Check sheet for the modelled part. Datum: model origin and axes. Units: mm. A direction names the side the tool comes from. Give positions to 0.01 mm unless a question says otherwise; leave off trailing zeros. Write each loop counter-clockwise with the first axis right and the second up, starting at its lowest first coordinate (ties: lowest second). Pieces come first, ordered by that corner, then holes. Notation, with made-up numbers: (40.5, 23) -> (99.5, 23) arc R30 cw to (99.5, 59) -> close; hole circle Ø2 at (0, 32). An arc over 180 degrees is marked (long way). Return JSON: item names as keys, results as strings.
from build123d import *

# Parameters (mm, degrees)
BOSS_EXTRUDE1_DEPTH = 9.05
SKETCH2_W           = 20
SKETCH2_H           = 10
CUT_EXTRUDE1_DEPTH  = 57.605743
FILLET1_R           = 3
SKETCH4_R           = 3
BOSS_EXTRUDE2_DEPTH = 0.95
CUT_EXTRUDE2_START  = -1.5
CUT_EXTRUDE2_DEPTH  = 1.5
SKETCH5_R           = 0.95
CUT_EXTRUDE3_DEPTH  = 57.765374


with BuildPart() as part:
    # Sketch1 → Boss-Extrude1 (new body)
    with BuildSketch(Plane.XY):
        with BuildLine():
            Line((-23.657, 29.8), (-23.657, 46.8))
            ThreePointArc((-23.657, 46.8), (-22.77832, 48.92132), (-20.657, 49.8))
            Line((-20.657, 49.8), (22.343, 49.8))
            ThreePointArc((22.343, 49.8), (24.46432, 48.92132), (25.343, 46.8))
            Line((25.343, 46.8), (25.343, 29.8))
            ThreePointArc((25.343, 29.8), (24.46432, 27.67868), (22.343, 26.8))
            Line((22.343, 26.8), (17.343, 26.8))
            ThreePointArc((17.343, 26.8), (15.22168, 25.92132), (14.343, 23.8))
            Line((14.343, 23.8), (14.343, -11.9))
            ThreePointArc((14.343, -11.9), (13.46432, -14.02132), (11.343, -14.9))
            Line((11.343, -14.9), (-9.657, -14.9))
            ThreePointArc((-9.657, -14.9), (-11.77832, -14.02132), (-12.657, -11.9))
            Line((-12.657, -11.9), (-12.657, 23.8))
            ThreePointArc((-12.657, 23.8), (-13.53568, 25.92132), (-15.657, 26.8))
            Line((-15.657, 26.8), (-20.657, 26.8))
            ThreePointArc((-20.657, 26.8), (-22.77832, 27.67868), (-23.657, 29.8))
        make_face()
    extrude(amount=BOSS_EXTRUDE1_DEPTH)

    # Sketch2 → Cut-Extrude1 (cut, through all)
    with BuildSketch(Plane.XY.offset(9.05)):
        with BuildLine():
            Line((-8.157, 11.8), (9.843, 11.8))
            ThreePointArc((9.843, 11.8), (10.550107, 12.092893), (10.843, 12.8))
            Line((10.843, 12.8), (10.843, 24.8))
            Line((10.843, 24.8), (-9.157, 24.8))
            Line((-9.157, 24.8), (-9.157, 12.8))
            ThreePointArc((-9.157, 12.8), (-8.864107, 12.092893), (-8.157, 11.8))
        make_face()
        with Locations((0.843, 29.8)):
            Rectangle(SKETCH2_W, SKETCH2_H)
    extrude(amount=-CUT_EXTRUDE1_DEPTH, mode=Mode.SUBTRACT)

    # Fillet1
    fillet1_edges = [part.edges().sort_by_distance(p)[0] for p in [
        (-9.157, 34.8, 4.525),
        (10.843, 34.8, 4.525),
    ]]
    fillet(fillet1_edges, radius=FILLET1_R)

    # Sketch4 → Boss-Extrude2 (add)
    with BuildSketch(Plane.XY.offset(9.05)):
        with Locations((22.343, 29.8)):
            Circle(SKETCH4_R)
        with Locations((22.343, 46.8)):
            Circle(SKETCH4_R)
        with Locations(Location((-20.657, 46.8, 0), (0, 0, 180))):
            Circle(SKETCH4_R)
        with Locations(Location((-20.657, 29.8, 0), (0, 0, 180))):
            Circle(SKETCH4_R)
    extrude(amount=BOSS_EXTRUDE2_DEPTH)

    # Sketch3 → Cut-Extrude2 (cut)
    with BuildSketch(Plane.XY.offset(9.05).offset(CUT_EXTRUDE2_START)):
        with BuildLine():
            Line((-12.657, 2.8), (14.343, 2.8))
            Line((14.343, 2.8), (14.343, 23.8))
            ThreePointArc((14.343, 23.8), (15.22168, 25.92132), (17.343, 26.8))
            Line((17.343, 26.8), (22.343, 26.8))
            ThreePointArc((22.343, 26.8), (20.22168, 31.92132), (25.343, 29.8))
            Line((25.343, 29.8), (25.343, 46.8))
            ThreePointArc((25.343, 46.8), (20.22168, 44.67868), (22.343, 49.8))
            Line((22.343, 49.8), (-20.657, 49.8))
            ThreePointArc((-20.657, 49.8), (-18.53568, 44.67868), (-23.657, 46.8))
            Line((-23.657, 46.8), (-23.657, 29.8))
            ThreePointArc((-23.657, 29.8), (-18.53568, 31.92132), (-20.657, 26.8))
            Line((-20.657, 26.8), (-15.657, 26.8))
            ThreePointArc((-15.657, 26.8), (-13.53568, 25.92132), (-12.657, 23.8))
            Line((-12.657, 23.8), (-12.657, 2.8))
        make_face()
        with BuildLine():
            Line((10.843, 31.8), (10.843, 12.8))
            ThreePointArc((10.843, 12.8), (10.550107, 12.092893), (9.843, 11.8))
            Line((9.843, 11.8), (-8.157, 11.8))
            ThreePointArc((-8.157, 11.8), (-8.864107, 12.092893), (-9.157, 12.8))
            Line((-9.157, 12.8), (-9.157, 31.8))
            ThreePointArc((-9.157, 31.8), (-8.27832, 33.92132), (-6.157, 34.8))
            Line((-6.157, 34.8), (7.843, 34.8))
            ThreePointArc((7.843, 34.8), (9.96432, 33.92132), (10.843, 31.8))
        make_face(mode=Mode.SUBTRACT)
    extrude(amount=CUT_EXTRUDE2_DEPTH, mode=Mode.SUBTRACT)

    # Sketch5 → Cut-Extrude3 (cut, through all)
    with BuildSketch(Plane.XY.offset(10)):
        with Locations((22.343, 46.8)):
            Circle(SKETCH5_R)
        with Locations((22.343, 29.8)):
            Circle(SKETCH5_R)
        with Locations((-20.657, 46.8)):
            Circle(SKETCH5_R)
        with Locations((-20.657, 29.8)):
            Circle(SKETCH5_R)
        with Locations((-9.657, -11.9)):
            Circle(SKETCH5_R)
        with Locations((11.343, -11.9)):
            Circle(SKETCH5_R)
        with Locations((11.343, 0.4)):
            Circle(SKETCH5_R)
        with Locations((0, 8.25)):
            Circle(SKETCH5_R)
        with Locations((-8.25, 0)):
            Circle(SKETCH5_R)
        with Locations((8.25, 0)):
            Circle(SKETCH5_R)
        with Locations((0, -8.25)):
            Circle(SKETCH5_R)
    extrude(amount=-CUT_EXTRUDE3_DEPTH, mode=Mode.SUBTRACT)


solid = part.part
(1) Release check for a two-part mould opening along Y. For faces 6 (the cylindrical face through (-20.78, 30.74, 5.07)), 7 (the flat face through (-22, 47, 10)), 8 (the cylindrical face through (-11.8, -14, 4.5)) record: pulls with the +Y half, pulls with the -Y half, needs draft (parallel to the pull), parting line crosses it, or undercut.
Reply:
{"face 6": "undercut", "face 7": "needs draft", "face 8": "pulls with the -Y half"}
(2) Set-up check for faces 1 (the flat face through (14.343, 6, 4)), 2 (the flat face through (-12.657, 6, 4)), 3 (the flat face through (1, -14.9, 4)), 4 (the cylindrical face through (9.941, 33.945, 3.722)), 5 (the flat face through (1, 2.8, 8)): record each of +Z, -Z, +X, -X, +Y, -Y from which the full face is reachable in a straight line by a thin tool's end or side.
Reply:
{"face 1": "+Z, -Z, +X, -Y", "face 2": "+Z, -Z, -X, -Y", "face 3": "+Z, -Z, +X, -X, -Y", "face 4": "+Z, -Z", "face 5": "+Z, +X, -X, +Y"}
(3) Thickness scan on L1, parallel to Y at x = -6, z = 4.75; L2, parallel to Y at x = 0, z = 4; L3, parallel to Y at x = 8.5, z = 3.25. Record the ranges inside material, lowest first.
Reply:
{"L1": "-14.9 to 11.8, 34.8 to 49.8", "L2": "-14.9 to -9.2, -7.3 to 7.3, 9.2 to 11.8, 34.8 to 49.8", "L3": "-14.9 to -0.92, 0.92 to 11.8, 34.73 to 49.8"}
(4) Cross-section at B-B on x = 6.5. Enter the section's corners in (y, z), then the cut area to 3 significant figures.
Reply:
{"outline": "(-14.9, 0) -> (11.8, 0) -> (11.8, 7.55) -> (2.8, 7.55) -> (2.8, 9.05) -> (-14.9, 9.05) -> close; (34.8, 0) -> (49.8, 0) -> (49.8, 7.55) -> (34.8, 7.55) -> close", "area": "341 mm^2"}
(5) Cross-section at C-C on x = 0. Enter the section's corners in (y, z), then the cut area to 3 significant figures.
Reply:
{"outline": "(-14.9, 0) -> (-9.2, 0) -> (-9.2, 9.05) -> (-14.9, 9.05) -> close; (-7.3, 0) -> (7.3, 0) -> (7.3, 7.55) -> (2.8, 7.55) -> (2.8, 9.05) -> (-7.3, 9.05) -> close; (9.2, 0) -> (11.8, 0) -> (11.8, 7.55) -> (9.2, 7.55) -> close; (34.8, 0) -> (49.8, 0) -> (49.8, 7.55) -> (34.8, 7.55) -> close", "area": "310 mm^2"}
(6) Cross-section at A-A on y = 8.25. Enter the section's corners in (x, z), then the cut area to 3 significant figures.
Reply:
{"outline": "(-12.66, 0) -> (-0.95, 0) -> (-0.95, 7.55) -> (-12.66, 7.55) -> close; (0.95, 0) -> (14.34, 0) -> (14.34, 7.55) -> (0.95, 7.55) -> close", "area": "190 mm^2"}
(7) Depth check by flat-ended pin: pin 1 Ø6 at (y, z) = (14, 3.5) entering from -X; pin 2 Ø14 at (x, y) = (-5.5, -6) entering from +Z; pin 3 Ø1.5 at (x, y) = (22.343, 29.8) entering from +Z; pin 4 Ø2 at (x, y) = (0, 8.25) entering from +Z. Enter the tip coordinate at first touch or a pass-through.
Reply:
{"pin 1": "x = -12.66", "pin 2": "z = 9.05", "pin 3": "through", "pin 4": "z = 7.55"}
(8) Cross-section at D-D on y = -8.25. Enter the section's corners in (x, z), then the cut area to 3 significant figures.
Reply:
{"outline": "(-12.66, 0) -> (-0.95, 0) -> (-0.95, 9.05) -> (-12.66, 9.05) -> close; (0.95, 0) -> (14.34, 0) -> (14.34, 9.05) -> (0.95, 9.05) -> close", "area": "227 mm^2"}
